The model under review builds one solid part; all positions refer to its coordinate system, in mm. A direction names the side the tool comes from. Coordinates: 2 decimals unless noted, no trailing zeros. Loops run counter-clockwise (first coordinate to the right, second up) from the corner with the lowest first, then second, coordinate; pieces in that order, holes last. Notation, with made-up numbers: (-21, -4) - (3, -4) arc R17 ccw to (3, 15) - close; hole circle Ø8 at (2.5, 43). An arc over 180 degrees is marked (long way). One line per item, written item: value. Start each with the question number.
1. To check wall thickness, follow line 1 (Y direction, x = 0, z = 3.45); line 2 (X direction, y = 1, z = 0.8); line 3 (X direction, y = 1.5, z = 2.2). State the ranges of each line that lie inside material, in increasing order.
2. Mouldability with a two-part tool opening along Y and no side actions: class faces 1 (the face through (-20, -3, 2)), 2 (the face through (12.72, -18.03, 2.54)), 3 (the face through (-1.3, -8.1, 5)) as +Y half, -Y half, draft (parallel to the pull), parting line (faces both ways), or undercut.
3. We need section A-A, the plane y = -18. Give the boundary of the cut face in (x, z).
4. Insertion check: P1, Ø3, axis at y = -16, z = 0.5, coming from the -X side; P2, Ø1.2, axis at x = -14.5, z = 1.5, coming from the -Y side; P3, Ø1.5, axis at x = -16.5, z = 3.5, coming from the +Y side. Each pin has a flat end and moves straight along its axis. Give the tip position at first contact, or say it passes through.
5. We need section B-B, the plane z = 2.8. Count the separate pieces of the cut face and the enclosed holes in it, then the cut area to 3 significant figures.
6. For faces 4 (the face through (14.026, 10.182, 2.465)), 5 (the face through (8.98, 17.55, 2.46)), 6 (the face through (-15, -3, 2)), list the 3-axis set-ups (+Z, -Z, +X, -X, +Y, -Y) from which the entire face can be reached by the end or side of a thin tool; tool diameter is ignored.
from build123d import *

# Parameters (mm, degrees)
F0_R     = 8
F1_DEPTH = 5
F2_R     = 2
F3_DEPTH = 25


with BuildPart() as f1:
    # F0 (on Top) → F1 (new body)
    with BuildSketch(Plane.XY):
        with BuildLine():
            ThreePointArc((-30.583005, -1), (-29.997219, -2.414214), (-28.583005, -3))
            Line((-28.583005, -3), (-12.328828, -3))
            ThreePointArc((-12.328828, -3), (-10.968, -3.402824), (-10.045712, -4.481481))
            ThreePointArc((-10.045712, -4.481481), (-9.04279, -6.263222), (-7.727447, -7.828573))
            Line((-7.727447, -7.828573), (11.608563, -26.91481))
            ThreePointArc((11.608563, -26.91481), (12.758948, -27.475161), (14.013553, -27.223484))
            Line((14.013553, -27.223484), (16.157528, -25.985659))
            ThreePointArc((16.157528, -25.985659), (17.08938, -24.771247), (16.889579, -23.253609))
            Line((16.889579, -23.253609), (8.76249, -9.177078))
            ThreePointArc((8.76249, -9.177078), (8.430932, -7.797155), (8.903933, -6.459101))
            ThreePointArc((8.903933, -6.459101), (9.945504, -4.699675), (10.643467, -2.777879))
            Line((10.643467, -2.777879), (17.504628, 23.510715))
            ThreePointArc((17.504628, 23.510715), (17.414713, 24.787153), (16.569452, 25.747835))
            Line((16.569452, 25.747835), (14.425477, 26.985659))
            ThreePointArc((14.425477, 26.985659), (12.907839, 27.18546), (11.693426, 26.253609))
            Line((11.693426, 26.253609), (3.566338, 12.177078))
            ThreePointArc((3.566338, 12.177078), (2.537068, 11.199979), (1.141779, 10.940582))
            ThreePointArc((1.141779, 10.940582), (-0.902714, 10.962897), (-2.91602, 10.606452))
            Line((-2.91602, 10.606452), (-29.113191, 3.404094))
            ThreePointArc((-29.113191, 3.404094), (-30.173661, 2.688008), (-30.583005, 1.475649))
            Line((-30.583005, 1.475649), (-30.583005, -1))
        make_face()
        with BuildLine():
            Line((6.866025, -9.892305), (14.657528, -23.387583))
            ThreePointArc((14.657528, -23.387583), (14.757428, -24.146402), (14.291503, -24.753609))
            Line((14.291503, -24.753609), (13.673617, -25.110345))
            ThreePointArc((13.673617, -25.110345), (13.046314, -25.236184), (12.471122, -24.956008))
            Line((12.471122, -24.956008), (0.043078, -12.688504))
            ThreePointArc((0.043078, -12.688504), (-0.190899, -11.626074), (0.683442, -10.978748))
            ThreePointArc((0.683442, -10.978748), (1.804868, -10.850919), (2.907292, -10.608848))
            ThreePointArc((2.907292, -10.608848), (4.238352, -10.150683), (5.5, -9.526279))
            ThreePointArc((5.5, -9.526279), (6.258819, -9.426379), (6.866025, -9.892305))
        make_face(mode=Mode.SUBTRACT)
        with BuildLine():
            ThreePointArc((-11.010106, 6.306945), (-9.973026, 5.97836), (-9.849596, 4.897495))
            ThreePointArc((-9.849596, 4.897495), (-10.708538, 2.515397), (-11, 0))
            ThreePointArc((-11, 0), (-11.292893, -0.707107), (-12, -1))
            Line((-12, -1), (-27.583005, -1))
            ThreePointArc((-27.583005, -1), (-28.290112, -0.707107), (-28.583005, 0))
            Line((-28.583005, 0), (-28.583005, 0.713473))
            ThreePointArc((-28.583005, 0.713473), (-28.378333, 1.319652), (-27.848098, 1.677696))
            Line((-27.848098, 1.677696), (-11.010106, 6.306945))
        make_face(mode=Mode.SUBTRACT)
        Circle(F0_R, mode=Mode.SUBTRACT)
        with BuildLine():
            Line((5.133975, 10.892305), (12.925477, 24.387583))
            ThreePointArc((12.925477, 24.387583), (13.532684, 24.853509), (14.291503, 24.753609))
            Line((14.291503, 24.753609), (14.909388, 24.396872))
            ThreePointArc((14.909388, 24.396872), (15.332019, 23.916531), (15.376976, 23.278312))
            Line((15.376976, 23.278312), (10.967028, 6.381559))
            ThreePointArc((10.967028, 6.381559), (10.163925, 5.647714), (9.166153, 6.081252))
            ThreePointArc((9.166153, 6.081252), (7.532667, 8.016167), (5.5, 9.526279))
            ThreePointArc((5.5, 9.526279), (5.034074, 10.133486), (5.133975, 10.892305))
        make_face(mode=Mode.SUBTRACT)
    extrude(amount=F1_DEPTH)

    # F2 (on face) → F3 (cut)
    with BuildSketch(Plane.XY.offset(5)):
        with Locations((-27, -4)):
            Circle(F2_R)
        with Locations((-22, -4)):
            Circle(F2_R)
        with Locations((-17, -4)):
            Circle(F2_R)
        with Locations((-12, -4)):
            Circle(F2_R)
        with Locations((9.464102, -8.392305)):
            Circle(F2_R)
        with Locations((11.964102, -12.722432)):
            Circle(F2_R)
        with Locations((16.964102, -21.382686)):
            Circle(F2_R)
        with Locations((14.464102, -17.052559)):
            Circle(F2_R)
        with Locations((2.535898, 12.392305)):
            Circle(F2_R)
        with Locations((5.035898, 16.722432)):
            Circle(F2_R)
        with Locations((10.035898, 25.382686)):
            Circle(F2_R)
        with Locations((7.535898, 21.052559)):
            Circle(F2_R)
    extrude(amount=-F3_DEPTH, mode=Mode.SUBTRACT)


solid = f1.part
Findings below:
1. line 1: -15.46 to -12.64, -11.31 to -8, 8 to 11
1. line 2: -30.58 to -28.54, -10.95 to -7.94, 7.94 to 11.63
1. line 3: -30.58 to -28.2, -10.9 to -7.86, 7.86 to 11.76
2. face 1: -Y half
2. face 2: undercut
2. face 3: draft
3. outline: (2.58, 0) - (5.42, 0) - (5.42, 5) - (2.58, 5) - close; (11.55, 0) - (12.7, 0) - (12.7, 5) - (11.55, 5) - close
4. P1: x = -0.97
4. P2: y = -3
4. P3: y = 7.08
5. separate pieces: 1
5. enclosed holes: 4
5. area: 430 mm2
6. face 4: +Z, -Z, +X
6. face 5: +Z, -Z
6. face 6: +Z, -Z, -X, -Y
